Design review of the part shown in the three views and the two pictorial views. Dimensions are in mm from the part's minimum x, y and z. A direction names the side the tool comes from. Round coordinates to 2 decimals unless told otherwise and drop trailing zeros. Write each loop counter-clockwise with the first axis right and the second up, starting at its lowest first coordinate (ties: lowest second). Pieces come first, ordered by that corner, then holes. Notation, with made-up numbers: (82.5, -27.75) - (141.5, -27.75) arc R36 ccw to (141.5, 9.25) - close; hole circle Ø6 at (-19, -7). An arc over 180 degrees is marked (long way). One line per item, written item: value. Start each with the question number.
Q1. Mouldability with a two-part tool opening along Z and no side actions: class the marked faces 4, 5 and 6 as +Z half, -Z half, draft (parallel to the pull), parting line (faces both ways), or undercut.
Q2. Clearance check with flat-ended pins moving along their axes: pin 1 Ø2 at (y, z) = (6, 8.5) entering from -X; pin 2 Ø1.5 at (x, y) = (3.5, 3.5) entering from +Z; pin 3 Ø1.5 at (x, y) = (2.5, 3) entering from -Z. State where each tip first meets the part, or that it passes through.
Q3. For probe 1 along Y at (x, z) = (2.65, 5); probe 2 along X at (y, z) = (8, 4.75); probe 3 along X at (y, z) = (7.25, 4.75), list the stretches that pass through material, from the lowest coordinate up.
Q4. Add section B-B on x = 1.3. Write out the cut boundary in (y, z), and give its area (3 significant figures).
Q5. Add section A-A on x = 3.45. Write out the cut boundary in (y, z).
Q6. Tool access review of the marked faces 1, 2 and 3: name each direction out of +Z, -Z, +X, -X, +Y, -Y from which nothing blocks a thin tool from reaching the whole face with its end or side.
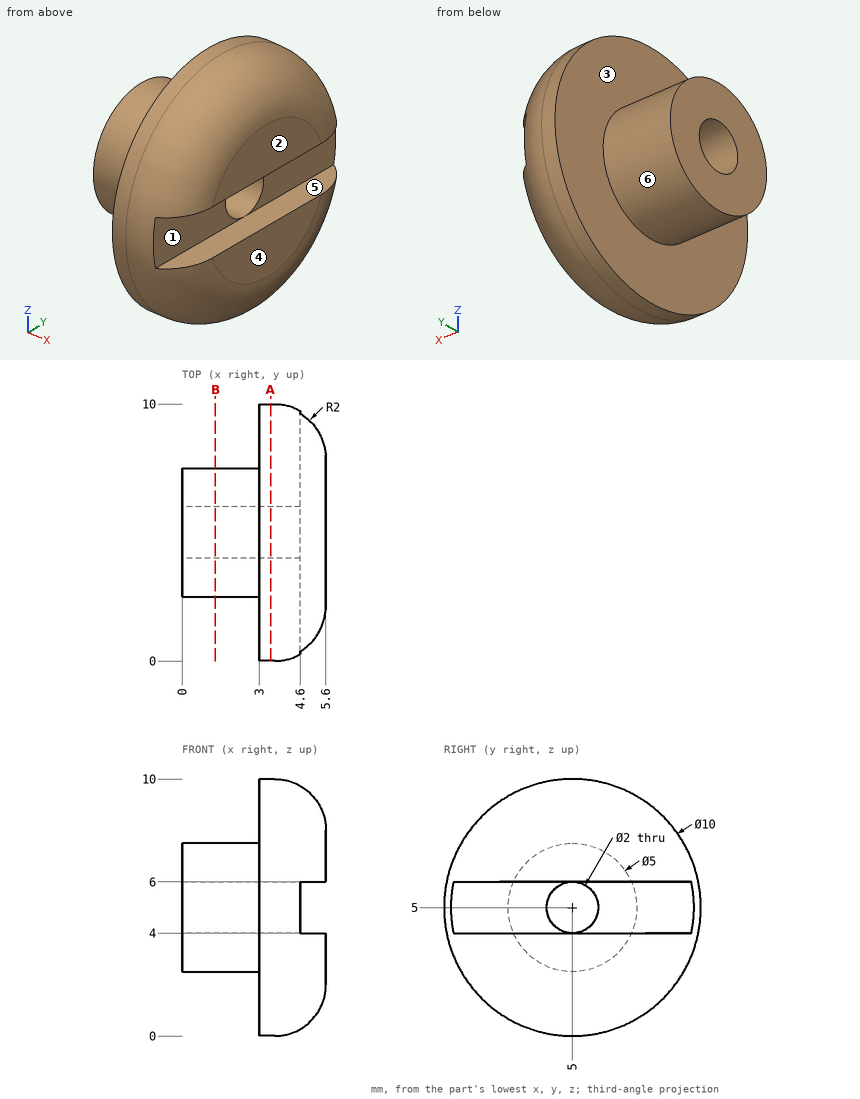
Result set:
1. face 4: draft
1. face 5: undercut
1. face 6: parting line
2. pin 1: stops at x = 3
2. pin 2: stops at z = 9.94
2. pin 3: stops at z = 0.21
3. probe 1: y = 2.5 to 4, 6 to 7.5
3. probe 2: x = 3 to 4.6
3. probe 3: x = 0 to 4.6
4. outline: circle Ø5 at (5, 5); hole circle Ø2 at (5, 5)
4. area: 16.5 mm^2
5. outline: circle Ø10 at (5, 5); hole circle Ø2 at (5, 5)
6. face 1: +X, +Y, -Y
6. face 2: +Z, -Z, +X, +Y, -Y
6. face 3: -X
